Build history of the part. All positions in model axes, mm. A direction names the side the tool comes from. Coordinates: 2 decimals unless noted, no trailing zeros. Order: outer loops, then holes, each group sorted by start corner. A loop starts at its lowest first (then second) coordinate and runs counter-clockwise, first axis right, second up. Notation, with made-up numbers: M -1.75,-1 L 3.25,-1 A27 cw 3.25,22 Z; hole C 71.25,75.25 d5. An arc over 180 degrees is marked long. Use a Markdown table: item, result. Add a question column.
from build123d import *

# Parameters (mm, degrees)
BOSS_EXTRUDE1_OUTLINE_R = 5
BOSS_EXTRUDE1_DEPTH     = 25
SKETCH3_W               = 4.1
SKETCH3_H               = 10.495866356
CUT_EXTRUDE1_DEPTH      = 8
CUT_EXTRUDE2_DEPTH      = 10


# Read off the part's stored shape, not the designer's step: Boss-Extrude1
with BuildPart() as part:
    # Boss-Extrude1 outline → Boss-Extrude1 (new body)
    with BuildSketch(Plane(origin=(0, 0, 0), x_dir=(1, 0, 0), z_dir=(0, 1, 0))):
        Circle(BOSS_EXTRUDE1_OUTLINE_R)
    extrude(amount=BOSS_EXTRUDE1_DEPTH)

    # Sketch3 → Cut-Extrude1 (cut)
    with BuildSketch(Plane(origin=(0, 25, 0), x_dir=(1, 0, 0), z_dir=(0, 1, 0))):
        Rectangle(SKETCH3_W, SKETCH3_H)
    extrude(amount=-CUT_EXTRUDE1_DEPTH, mode=Mode.SUBTRACT)

    # Sketch2 → Cut-Extrude2 (cut)
    with BuildSketch(Plane.XZ):
        with BuildLine():
            Line((-2.3, 2.003122562), (-2.3, -2.003122562))
            ThreePointArc((-2.3, -2.003122562), (0, -3.05), (2.3, -2.003122562))
            Line((2.3, -2.003122562), (2.3, 2.003122562))
            ThreePointArc((2.3, 2.003122562), (0, 3.05), (-2.3, 2.003122562))
        make_face()
    extrude(amount=-CUT_EXTRUDE2_DEPTH, mode=Mode.SUBTRACT)


solid = part.part
(1) Mould opens along X. For faces 4 (the cylindrical face through (4.77, 12.32, -1.5)), 5 (the flat face through (-3, 25, 0)), 6 (the cylindrical face through (-0.04, 4.93, -3.05)) say: released by +X, released by -X, zero draft, split by the parting line, or undercut.
(2) Drop flat-ended pins along their axis: P1, Ø2, axis at x = 3, y = 4.5, coming from the -Z side; P2, Ø1.4, axis at x = 0.5, z = -1.5, coming from the -Y side. Give the stop position or say it passes through.
(3) Drill centre lines: line 1 along X through (y, z) = (18.75, -0.25); line 2 along Y through (x, z) = (-1.25, 1.25); line 3 along X through (y, z) = (21.25, -3). Where is each one in solid material? Low to high. Write a range as from..to.
(4) Which spindle directions (+Z, -Z, +X, -X, +Y, -Y) get a long thin tool onto all of the face, cutting with end or side? Do faces 1 (the flat face through (0, 17, 0)), 2 (the flat face through (3, 25, 0)), 3 (the cylindrical face through (0.04, 4.93, 3.05)). Say none if no direction does.
(5) Slice it at A-A on z = 0. Give the cut face in (x, y), and give its area (3 significant figures).
(6) Slice it at C-C on y = 22.5. Give the cut face in (x, z), and give its area (3 significant figures).
(7) Slice it at B-B on x = 0. Give the cut face in (y, z), and give its area (3 significant figures).
(8) Slice it at D-D on y = 8. Give the cut face in (x, z).
Solutions:
| question | item | result |
|---|---|---|
| 1 | face 4 | split by the parting line |
| 1 | face 5 | zero draft |
| 1 | face 6 | undercut |
| 2 | P1 | z = -4.58 |
| 2 | P2 | y = 10 |
| 3 | line 1 | -4.99..-2.05, 2.05..4.99 |
| 3 | line 2 | 10..17 |
| 3 | line 3 | -4..-2.05, 2.05..4 |
| 4 | face 1 | +Z, -Z, +Y |
| 4 | face 2 | +Z, -Z, +X, -X, +Y |
| 4 | face 3 | -Y |
| 5 | outline | M -5,0 L -2.3,0 L -2.3,10 L 2.3,10 L 2.3,0 L 5,0 L 5,25 L 2.05,25 L 2.05,17 L -2.05,17 L -2.05,25 L -5,25 Z |
| 5 | area | 171 mm² |
| 6 | outline | M -2.05,-4.56 L -2.05,4.56 A5 ccw Z; M 2.05,-4.56 A5 ccw 2.05,4.56 Z |
| 6 | area | 38.7 mm² |
| 7 | outline | M 0,-5 L 17,-5 L 17,5 L 0,5 L 0,3.05 L 10,3.05 L 10,-3.05 L 0,-3.05 Z |
| 7 | area | 109 mm² |
| 8 | outline | C 0,0 d10; hole M -2.3,-2 A3.05 ccw 2.3,-2 L 2.3,2 A3.05 ccw -2.3,2 Z |
